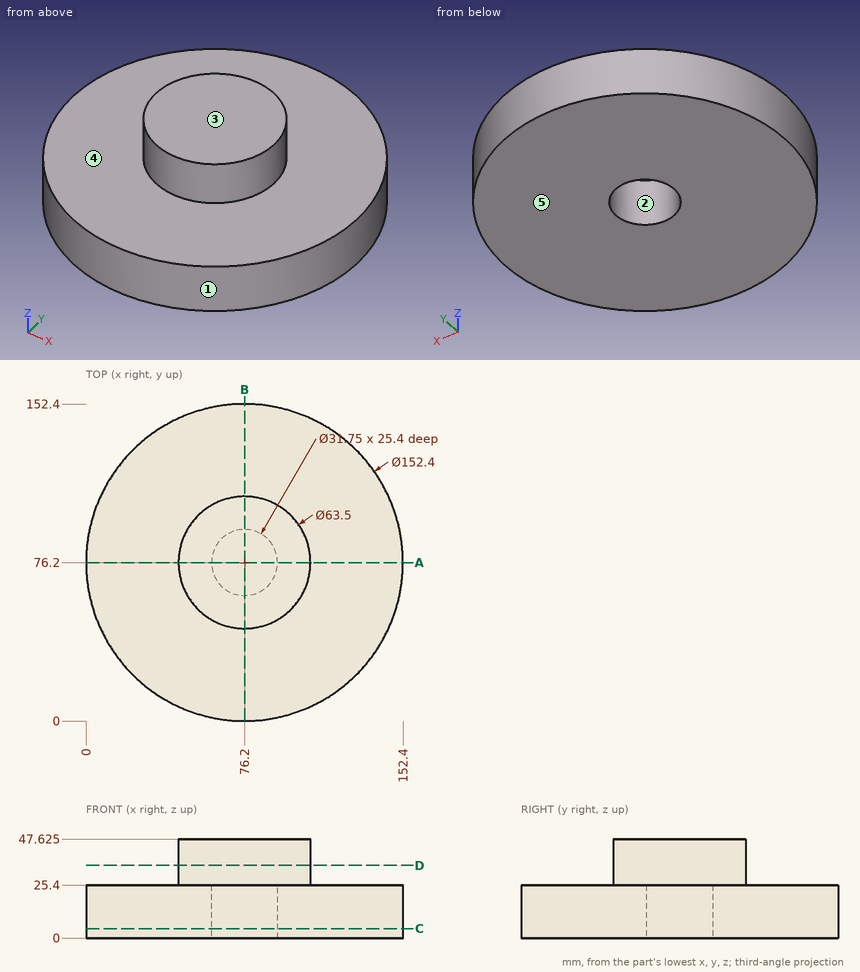
Check sheet for the drawn part. Datum: minimum x, y, z corner. Units: mm. A direction names the side the tool comes from. Give positions to 0.01 mm unless a question says otherwise; leave off trailing zeros. Order: outer loops, then holes, each group sorted by start corner. A loop starts at its lowest first (then second) coordinate and runs counter-clockwise, first axis right, second up.
1. Access from +Z, -Z, +X, -X, +Y, -Y to the whole of each face (thin tool, end or side, straight path). Record for the marked faces 4 and 5.
Completed:
face 4: +Z
face 5: -Z, +X, -X, +Y, -Y
2. Sectioned sample at D-D (z = 35). Record the boundary of the cut face in (x, y), then the cut area to 3 significant figures.
Completed:
outline: circle Ø63.5 at (76.2, 76.2)
area: 3,170 mm2
3. Draft check along X on the marked faces 1, 2 and 3. Enter one of: pulls with the +X half, pulls with the -X half, needs draft (parallel to the pull), parting line crosses it, or undercut.
Completed:
face 1: parting line crosses it
face 2: undercut
face 3: needs draft
4. Sectioned sample at C-C (z = 4.5). Record the boundary of the cut face in (x, y) (3 decimals).
Completed:
outline: circle Ø152.4 at (76.2, 76.2); hole circle Ø31.75 at (76.2, 76.2)
5. Scan lines: line 1 (Y direction, x = 76, z = 16); line 2 (Z direction, x = 30.5, y = 27). Record each from-to range of solid material in increasing order.
Completed:
line 1: y = 0 to 60.33, 92.07 to 152.4
line 2: z = 0 to 25.4
6. Depth check by flat-ended pin: pin 1 (16 mm diameter, centred on x = 78, y = 72.5, fed in from -Z); pin 2 (5 mm diameter, centred on x = 118, y = 132, fed in from +Z); pin 3 (5 mm diameter, centred on x = 64.5, z = 33.5, fed in from +Y). Enter the tip coordinate at first touch or a pass-through.
Completed:
pin 1: stops at z = 25.4
pin 2: stops at z = 25.4
pin 3: stops at y = 106.59
7. Sectioned sample at A-A (y = 76.2). Record the boundary of the cut face in (x, z) (3 decimals), then the cut area to 3 significant figures.
Completed:
outline: (0, 0) - (60.325, 0) - (60.325, 25.4) - (92.075, 25.4) - (92.075, 0) - (152.4, 0) - (152.4, 25.4) - (107.95, 25.4) - (107.95, 47.625) - (44.45, 47.625) - (44.45, 25.4) - (0, 25.4) - close
area: 4,480 mm2
